Autodesk Fusion 360 part; units mm, degrees
sketch "Skizze1" plane through (0, 0, 0) normal (0, 0, 1) x (1, 0, 0)
  line L0 (0, 0) -> (127, 0)
  line L1 (127, 0) -> (127, 143.5)
  line L2 (127, 143.5) -> (0, 143.5)
  line L3 (0, 143.5) -> (0, 0)
  line L4 (98, 50) -> (58, 50)
  line L5 (58, 50) -> (58, 9)
  line L6 (58, 9) -> (98, 9)
  line L7 (98, 9) -> (98, 50)
  circle A0 centre (84.6667, 4.5) radius 1.5
  circle A1 centre (42.3337, 4.5) radius 1.5
  dimension "d1" = 127
  dimension "d2" = 143.5
  dimension "d3" = 40
  dimension "d4" = 29
  dimension "d5" = 50
  dimension "d6" = 41
  dimension "d7" = 3
  dimension "d8" = 4.5
  dimension "d9" = 42.3333
  dimension "d10" = 3
extrude "Extrusion1" add sketch "Skizze1" along normal blind 9
equation "d5 = 41 mm + 9 mm"
equation "d8 = ( 9 / 2 ) * 1 mm"
equation "d9 = ( 127 / 3 ) * 1 mm"
Model file for the job. Use its own axes, mm. A direction names the side the tool comes from. Give positions to 0.01 mm unless a question says otherwise; leave off trailing zeros. Write each loop counter-clockwise with the first axis right and the second up, starting at its lowest first coordinate (ties: lowest second). Pieces come first, ordered by that corner, then holes. Notation, with made-up numbers: (84.25, 8) -> (139.25, 8) arc R15 cw to (139.25, 28) -> close; hole circle Ø11 at (50, -30.75). An arc over 180 degrees is marked (long way). Write item = value, one per line.
(1) Flat gauge pin, fed straight in: P1, Ø2.5, axis at x = 84.67, y = 4.5, coming from the -Z side. Where does the tip first touch, or does it go through?
Determined:
P1 = through
(2) Slice it at B-B, the plane x = 79. Give the cut face in (y, z).
Determined:
outline = (0, 0) -> (9, 0) -> (9, 9) -> (0, 9) -> close; (50, 0) -> (143.5, 0) -> (143.5, 9) -> (50, 9) -> close
(3) Slice it at C-C, the plane z = 3.75. Give the cut face in (x, y).
Determined:
outline = (0, 0) -> (127, 0) -> (127, 143.5) -> (0, 143.5) -> close; hole circle Ø3 at (42.33, 4.5); hole (58, 9) -> (98, 9) -> (98, 50) -> (58, 50) -> close; hole circle Ø3 at (84.67, 4.5)
(4) Mould opens along Y. For faces 1 (the face through (64, 143.5, 4)), 2 (the face through (43.764, 4.049, 4.437)), 3 (the face through (127, 71, 4)) say: released by +Y, released by -Y, zero draft, split by the parting line, or undercut.
Determined:
face_1 = released by +Y
face_2 = undercut
face_3 = zero draft
(5) Tool access for faces 4 (the face through (78, 50, 4)), 5 (the face through (0, 73, 4)): list every direction of +Z, -Z, +X, -X, +Y, -Y with a clear straight run to the whole face (end or side of a thin tool).
Determined:
face_4 = +Z, -Z
face_5 = +Z, -Z, -X, +Y, -Y
(6) Slice it at A-A, the plane y = 20. Give the cut face in (x, z), then the cut area to 3 significant figures.
Determined:
outline = (0, 0) -> (58, 0) -> (58, 9) -> (0, 9) -> close; (98, 0) -> (127, 0) -> (127, 9) -> (98, 9) -> close
area = 783 mm2
(7) Probe line 1 along Y through (x, z) = (67, 1.5); line 2 along X through (y, z) = (9.5, 6). List the from-to ranges inside material, lowest first.
Determined:
line_1 = 0 to 9, 50 to 143.5
line_2 = 0 to 58, 98 to 127
